The listing builds one solid part. Answer for the finished solid, in the listing's coordinates (mm). Face numbers are marked on the shaded views. Round coordinates to 2 decimals unless told otherwise and drop trailing zeros. Loops run counter-clockwise (first coordinate to the right, second up) from the corner with the lowest first, then second, coordinate; pieces in that order, holes last. Notation, with made-up numbers: (-20, 82) -> (16, 82) arc R21 ccw to (16, 110) -> close; hole circle Ø10 at (47.5, 49.5). An arc over 180 degrees is marked (long way). Write each question's results on one line, items separated by ' | '. Start each with the question number.
(1) The part is cut by section A-A (y = -37.5). Determine the outline of the cut face in (x, z), plus the area to 3 significant figures.
(2) Straight lines are drawn through the part: probe 1 along Z at (x, y) = (0, -9); probe 2 along X at (y, z) = (-17, -6); probe 3 along Y at (x, z) = (23, 23). For each, find the intervals that lie inside material, in ascending order.
(3) Flat-ended cylindrical pins translate along their axes: pin 1 (10 mm diameter, centred on x = 54, z = -12, fed in from -Y); pin 2 (12 mm diameter, centred on y = -14, z = -6, fed in from -X); pin 3 (6 mm diameter, centred on x = -5, y = -21, fed in from +Z). Find the tip coordinate at first contact, or state that the pin passes through.
(4) Determine the mould class of the marked faces 1, 2 and 3 for opening direction X: released by +X, released by -X, zero draft, split by the parting line, or undercut.
(5) The part is cut by section B-B (z = 6). Count the separate pieces of the cut face and the enclosed holes in it, plus the area to 3 significant figures.
```python
from build123d import *

# Parameters (mm, degrees)
F0_R     = 15
F0_R_2   = 10
F1_DEPTH = 25
F2_DEPTH = 50
F3_R     = 2
F4_SIZE  = 3


# Not quite as in the source:
# - a feature names something its author has since deleted; it is built from what else it names


with BuildPart() as f1:
    # F0 (on Front) → F1 (new body)
    with BuildSketch(Plane.XZ):
        with BuildLine():
            ThreePointArc((6.25, -29.3417364858), (23.3184476327, -18.8745860882), (30, 0))
            ThreePointArc((30, 0), (23.3184476327, 18.8745860882), (6.25, 29.3417364858))
            ThreePointArc((6.25, 29.3417364858), (-30, 0), (6.25, -29.3417364858))
        make_face()
        Circle(F0_R, mode=Mode.SUBTRACT)
        with BuildLine():
            ThreePointArc((6.25, 29.3417364858), (23.3184476327, 18.8745860882), (30, 0))
            ThreePointArc((30, 0), (23.3184476327, -18.8745860882), (6.25, -29.3417364858))
            Line((6.25, -29.3417364858), (63.6458333333, -17.11601295))
            ThreePointArc((63.6458333333, -17.11601295), (42.5, 0), (63.6458333333, 17.11601295))
            Line((63.6458333333, 17.11601295), (6.25, 29.3417364858))
        make_face()
        with BuildLine():
            ThreePointArc((77.5, 0), (73.6024277858, 11.0101752181), (63.6458333333, 17.11601295))
            ThreePointArc((63.6458333333, 17.11601295), (42.5, 0), (63.6458333333, -17.11601295))
            ThreePointArc((63.6458333333, -17.11601295), (73.6024277858, -11.0101752181), (77.5, 0))
        make_face()
        with Locations((60, 0)):
            Circle(F0_R_2, mode=Mode.SUBTRACT)
    extrude(amount=F1_DEPTH)

    # F0 (on Front) → F2 (join)
    with BuildSketch(Plane.XZ):
        with BuildLine():
            ThreePointArc((6.25, -29.3417364858), (23.3184476327, -18.8745860882), (30, 0))
            ThreePointArc((30, 0), (23.3184476327, 18.8745860882), (6.25, 29.3417364858))
            ThreePointArc((6.25, 29.3417364858), (-30, 0), (6.25, -29.3417364858))
        make_face()
        Circle(F0_R, mode=Mode.SUBTRACT)
    extrude(amount=F2_DEPTH)

    # F3
    f3_edges = [f1.edges().sort_by_distance(p)[0] for p in [
        (-6.25, -50, 29.341736),
        (34.947917, 0, -23.228875),
    ]]
    fillet(f3_edges, radius=F3_R)

    # F4
    f4_edges = [f1.edges().sort_by_distance(p)[0] for p in [
        (-15, -50, 0),
        (70, -12.5, 0),
        (50, 0, 0),
        (50, -25, 0),
    ]]
    chamfer(f4_edges, length=F4_SIZE)


solid = f1.part
```
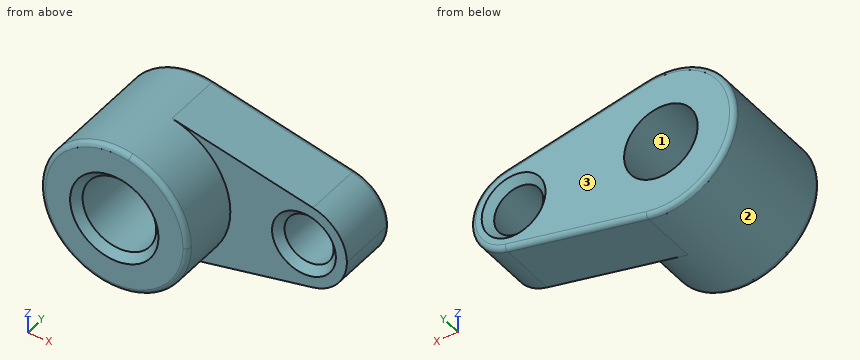
Checked values:
1) outline: circle Ø60 at (0, 0); hole circle Ø30 at (0, 0) | area: 2,120 mm2
2) probe 1: z = -30 to -15, 15 to 30 | probe 2: x = -29.39 to -13.75, 13.75 to 52, 68 to 76.44 | probe 3: y = -25 to 0
3) pin 1: stops at y = -25 | pin 2: stops at x = -30 | pin 3: stops at z = 29.93
4) face 1: undercut | face 2: split by the parting line | face 3: zero draft
5) separate pieces: 3 | enclosed holes: 0 | area: 2,310 mm2
